```python
from build123d import *

# Parameters (mm, degrees)
SKETCH1_W           = 24
SKETCH1_H           = 25
SKETCH1_R           = 1.125
BOSS_EXTRUDE1_DEPTH = 3
BOSS_EXTRUDE2_DEPTH = 8


with BuildPart() as part:
    # Sketch1 → Boss-Extrude1 (new body)
    with BuildSketch(Plane.XY):
        Rectangle(SKETCH1_W, SKETCH1_H)
        with Locations((-6.75, 6.55)):
            Circle(SKETCH1_R, mode=Mode.SUBTRACT)
        with Locations((-6.75, -0.25)):
            Circle(SKETCH1_R, mode=Mode.SUBTRACT)
        with Locations((-6.75, -7.05)):
            Circle(SKETCH1_R, mode=Mode.SUBTRACT)
        with Locations((6.75, -7.05)):
            Circle(SKETCH1_R, mode=Mode.SUBTRACT)
        with Locations((6.75, -0.25)):
            Circle(SKETCH1_R, mode=Mode.SUBTRACT)
        with Locations((6.75, 6.55)):
            Circle(SKETCH1_R, mode=Mode.SUBTRACT)
    extrude(amount=BOSS_EXTRUDE1_DEPTH)

    # Sketch2 → Boss-Extrude2 (add)
    with BuildSketch(Plane.XY):
        Polygon((-12, 12.5), (-15, 12.5), (-15, -12.5), (-12, -12.5), (-12, -10.882685902), (-8.625, -8.934128744), (-12, -6.985571585), (-8.625, -5.037014427), (-12, -3.088457268), (-8.625, -1.13990011), (-12, 0.808657049), (-8.625, 2.757214207), (-12, 4.705771366), (-8.625, 6.654328524), (-12, 8.602885683), (-8.625, 10.551442841), align=None)
        Polygon((12, -3.088457268), (8.625, -5.037014427), (12, -6.985571585), (8.625, -8.934128744), (12, -10.882685902), (12, -12.5), (15, -12.5), (15, 12.5), (12, 12.5), (8.625, 10.551442841), (12, 8.602885683), (8.625, 6.654328524), (12, 4.705771366), (8.625, 2.757214207), (12, 0.808657049), (8.625, -1.13990011), align=None)
    extrude(amount=BOSS_EXTRUDE2_DEPTH)


solid = part.part
```
Here's how the part is built. I have some questions about the finished solid (model axes, mm). A direction names the side the tool comes from. Round coordinates to 2 decimals unless told otherwise and drop trailing zeros. Order: outer loops, then holes, each group sorted by start corner. A loop starts at its lowest first (then second) coordinate and runs counter-clockwise, first axis right, second up. Notation, with made-up numbers: M 24.5,22 L 29.5,22 A31 cw 29.5,56 Z; hole C 0,79 d7. An arc over 180 degrees is marked long. Answer as CSV lines item,"result".
Item 1: Which directions (+Z, -Z, +X, -X, +Y, -Y) give clear straight access to the entire face, cutting with the end or side of a thin tool? Please do faces 4 (the cylindrical face through (-6.231, 5.552, 1.479)), 5 (the flat face through (12, 0, 8)), 6 (the flat face through (-10.289, -4.076, 5.465)), 7 (the flat face through (10.34, 11.54, 5.46)), 8 (the flat face through (-10.3, -9.9, 5.5)).
From the geometry:
face 4,"+Z, -Z"
face 5,"+Z, +X, -X, +Y, -Y"
face 6,"+Z"
face 7,"+Z, +Y"
face 8,"+Z, -Y"
Item 2: Imagine slicing it at C-C on y = -0.75. List the corners of the cut face in (x, z) for me.
From the geometry:
outline,"M -15,0 L -7.76,0 L -7.76,3 L -9.3,3 L -9.3,8 L -15,8 Z; M -5.74,0 L 5.74,0 L 5.74,3 L -5.74,3 Z; M 7.76,0 L 15,0 L 15,8 L 9.3,8 L 9.3,3 L 7.76,3 Z"
Item 3: Please list where these lines run through material, in increasing order: L1, parallel to Y at x = -6.75, z = 2.4 (3 decimals); L2, parallel to Y at x = -10.25, z = 6.5; L3, parallel to Y at x = -10, z = 5.75. Write a range as [from, to].
From the geometry:
L1,"[-12.5, -8.175], [-5.925, -1.375], [0.875, 5.425], [7.675, 12.5]"
L2,"[-9.87, -8], [-5.98, -4.1], [-2.08, -0.2], [1.82, 3.7], [5.72, 7.59], [9.61, 11.49]"
L3,"[-9.73, -8.14], [-5.83, -4.24], [-1.93, -0.35], [1.96, 3.55], [5.86, 7.45], [9.76, 11.35]"
Item 4: Imagine slicing it at D-D on z = 2. List the corners of the cut face in (x, y) for me (3 decimals).
From the geometry:
outline,"M -15,-12.5 L 15,-12.5 L 15,12.5 L -15,12.5 Z; hole C -6.75,-7.05 d2.25; hole C -6.75,-0.25 d2.25; hole C -6.75,6.55 d2.25; hole C 6.75,-7.05 d2.25; hole C 6.75,-0.25 d2.25; hole C 6.75,6.55 d2.25"
Item 5: Imagine slicing it at B-B on x = -6.75. List the corners of the cut face in (y, z) for me (3 decimals).
From the geometry:
outline,"M -12.5,0 L -8.175,0 L -8.175,3 L -12.5,3 Z; M -5.925,0 L -1.375,0 L -1.375,3 L -5.925,3 Z; M 0.875,0 L 5.425,0 L 5.425,3 L 0.875,3 Z; M 7.675,0 L 12.5,0 L 12.5,3 L 7.675,3 Z"
Item 6: For pin 1 (3.5 mm diameter, centred on x = 6.75, y = 6.55, fed in from +Z); pin 2 (2 mm diameter, centred on x = 6.75, y = -0.25, fed in from -Z), each with a flat end and sliding along its axis, tell me the tip position at first contact or that it passes through.
From the geometry:
pin 1,"z = 3"
pin 2,"through"
Item 7: We'd pull the mould along Y, two halves only. Please class faces 1 (the flat face through (-10.289, 11.512, 5.465)), 2 (the flat face through (-10.29, -0.18, 5.46)), 3 (the flat face through (-12, -12, 5)): +Y half, -Y half, draft (parallel to the pull), parting line (faces both ways), or undercut.
From the geometry:
face 1,"+Y half"
face 2,"undercut"
face 3,"draft"
